from build123d import *

# Parameters (mm, degrees)
SKETCH1_W           = 59
SKETCH1_H           = 52
BOSS_EXTRUDE1_DEPTH = 5.5
SKETCH2_R           = 2
CUT_EXTRUDE1_DEPTH  = 10
SKETCH4_W           = 7
SKETCH4_H           = 52
BOSS_EXTRUDE3_DEPTH = 40
SKETCH5_R           = 2.5
CUT_EXTRUDE2_DEPTH  = 33
SKETCH6_W           = 13.8
SKETCH6_H           = 40
CUT_EXTRUDE3_DEPTH  = 33
CUT_EXTRUDE4_DEPTH  = 33
BOSS_EXTRUDE6_DEPTH = 38.2
SKETCH10_W          = 13
SKETCH10_H          = 9
CUT_EXTRUDE8_DEPTH  = 10
SKETCH11_R          = 11.5
CUT_EXTRUDE9_DEPTH  = 10


with BuildPart() as part:
    # Sketch1 → Boss-Extrude1 (new body)
    with BuildSketch(Plane(origin=(0, 0, 0), x_dir=(1, 0, 0), z_dir=(0, 1, 0))):
        with Locations((-29.5, -26)):
            Rectangle(SKETCH1_W, SKETCH1_H)
    extrude(amount=BOSS_EXTRUDE1_DEPTH)

    # Sketch2 → Cut-Extrude1 (cut)
    with BuildSketch(Plane(origin=(0, 5.5, 0), x_dir=(1, 0, 0), z_dir=(0, 1, 0))):
        with Locations(Location((-53.6, -5.4, 0), (0, 0, 270))):
            Circle(SKETCH2_R)
        with Locations(Location((-22.6, -5.4, 0), (0, 0, 270))):
            Circle(SKETCH2_R)
        with Locations(Location((-53.6, -36.5, 0), (0, 0, 270))):
            Circle(SKETCH2_R)
        with Locations(Location((-22.6, -36.5, 0), (0, 0, 270))):
            Circle(SKETCH2_R)
    extrude(amount=-CUT_EXTRUDE1_DEPTH, mode=Mode.SUBTRACT)

    # Sketch4 → Boss-Extrude3 (add)
    with BuildSketch(Plane(origin=(0, 0, 0), x_dir=(-1, 0, 0), z_dir=(0, -1, 0))):
        with Locations((3.5, -26)):
            Rectangle(SKETCH4_W, SKETCH4_H)
    extrude(amount=BOSS_EXTRUDE3_DEPTH)

    # Sketch5 → Cut-Extrude2 (cut)
    with BuildSketch(Plane.ZY.offset(7)):
        with Locations((43.8, -32.7)):
            Circle(SKETCH5_R)
        with Locations((43.8, -12.7)):
            Circle(SKETCH5_R)
        with Locations((23.8, -32.7)):
            Circle(SKETCH5_R)
        with Locations((23.8, -12.7)):
            Circle(SKETCH5_R)
    extrude(amount=-CUT_EXTRUDE2_DEPTH, mode=Mode.SUBTRACT)

    # Sketch6 → Cut-Extrude3 (cut)
    with BuildSketch(Plane.ZY.offset(7)):
        with Locations((6.9, -20)):
            Rectangle(SKETCH6_W, SKETCH6_H)
    extrude(amount=-CUT_EXTRUDE3_DEPTH, mode=Mode.SUBTRACT)

    # Sketch7 → Cut-Extrude4 (cut)
    with BuildSketch(Plane(origin=(0, 0, 0), x_dir=(-1, 0, 0), z_dir=(0, -1, 0))):
        Polygon((0, 0), (0, -13.8), (17.836375114, 0), align=None)
    extrude(amount=-CUT_EXTRUDE4_DEPTH, mode=Mode.SUBTRACT)

    # Sketch8 → Boss-Extrude6 (add)
    with BuildSketch(Plane.XY.offset(52)):
        Polygon((-7, 0), (-7, -8), (-17, 0), align=None)
    extrude(amount=-BOSS_EXTRUDE6_DEPTH)

    # Sketch10 → Cut-Extrude8 (cut)
    with BuildSketch(Plane.ZY.offset(7)):
        with Locations((24.3, -22.7)):
            Rectangle(SKETCH10_W, SKETCH10_H)
    extrude(amount=-CUT_EXTRUDE8_DEPTH, mode=Mode.SUBTRACT)

    # Sketch11 → Cut-Extrude9 (cut)
    with BuildSketch(Plane(origin=(0, 5.5, 0), x_dir=(1, 0, 0), z_dir=(0, 1, 0))):
        with Locations(Location((-38.1, -21, 0), (0, 0, 270))):
            Circle(SKETCH11_R)
    extrude(amount=-CUT_EXTRUDE9_DEPTH, mode=Mode.SUBTRACT)


solid = part.part
The model under review builds one solid part; all positions refer to its coordinate system, in mm. A direction names the side the tool comes from. Coordinates: 2 decimals unless noted, no trailing zeros. Loops run counter-clockwise (first coordinate to the right, second up) from the corner with the lowest first, then second, coordinate; pieces in that order, holes last. Notation, with made-up numbers: M 89.5,79 L 96.5,79 A7 cw 96.5,90 Z; hole C 35.25,-18.75 d5. An arc over 180 degrees is marked long. Put each result on its own line as item: value. Start each with the question number.
Q1. Add section A-A (x = -53.6). Write out the cut boundary in (y, z), and give its area (3 significant figures).
Q2. Clearance check with flat-ended pins moving along their axes: pin 1 (6.5 mm diameter, centred on x = -53.6, z = 5.4, fed in from -Y); pin 2 (6 mm diameter, centred on y = -22.5, z = 13, fed in from -X); pin 3 (3 mm diameter, centred on y = -3, z = 25.5, fed in from -X) (3 decimals). State where each tip first meets the part, or that it passes through.
Q3. For faces 4 (the flat face through (-7, -24, 33)), 5 (the cylindrical face through (-55.374, 2.788, 37.423)), list the 3-axis set-ups (+Z, -Z, +X, -X, +Y, -Y) from which the entire face can be reached by the end or side of a thin tool; tool diameter is ignored.
Q4. Add section C-C (z = 16). Write out the cut boundary in (x, y).
Q5. Add section B-B (y = -21.5). Write out the cut boundary in (x, z).
Q6. The part is to be moulded in two halves that separate along Z. For faces 1 (the flat face through (-4, -27.2, 24)), 2 (the flat face through (0, -17, 33)), 3 (the flat face through (-38, 3, 0)), say which applies: +Z half, -Z half, draft (parallel to the pull), parting line (faces both ways), or undercut.
Q7. Wall thickness on line 1 (X direction, y = 1.4, z = 36.5); line 2 (Y direction, x = -2.75, z = 23.8); line 3 (Y direction, x = -3, z = 43): over which ranges is each line inside the solid? List them lowest first.
Q8. Add section D-D (z = 33.5). Write out the cut boundary in (x, y), and give its area (4 significant figures).
Answers:
1. outline: M 0,0 L 5.5,0 L 5.5,3.4 L 0,3.4 Z; M 0,7.4 L 5.5,7.4 L 5.5,34.5 L 0,34.5 Z; M 0,38.5 L 5.5,38.5 L 5.5,52 L 0,52 Z
1. area: 242 mm^2
2. pin 1: stops at y = 0
2. pin 2: stops at x = -7
2. pin 3: stops at x = -15.125
3. face 4: +Z, -Z, -X, -Y
3. face 5: +Y, -Y
4. outline: M -59,0 L -48.46,0 L -48.46,5.5 L -59,5.5 Z; M -27.74,0 L -17,0 L -7,-8 L -7,-40 L 0,-40 L 0,5.5 L -27.74,5.5 Z
5. outline: M -7,13.8 L 0,13.8 L 0,17.8 L -7,17.8 Z; M -7,30.8 L 0,30.8 L 0,52 L -7,52 Z
6. face 1: undercut
6. face 2: draft
6. face 3: -Z half
7. line 1: x = -59 to -55.6, -51.6 to -24.6, -20.6 to 0
7. line 2: y = -40 to -35.2, -30.2 to -27.2, -18.2 to -15.2, -10.2 to 5.5
7. line 3: y = -40 to -35.07, -30.33 to -15.07, -10.33 to 5.5
8. outline: M -59,0 L -17,0 L -7,-8 L -7,-40 L 0,-40 L 0,5.5 L -59,5.5 Z
8. area: 644.5 mm^2
